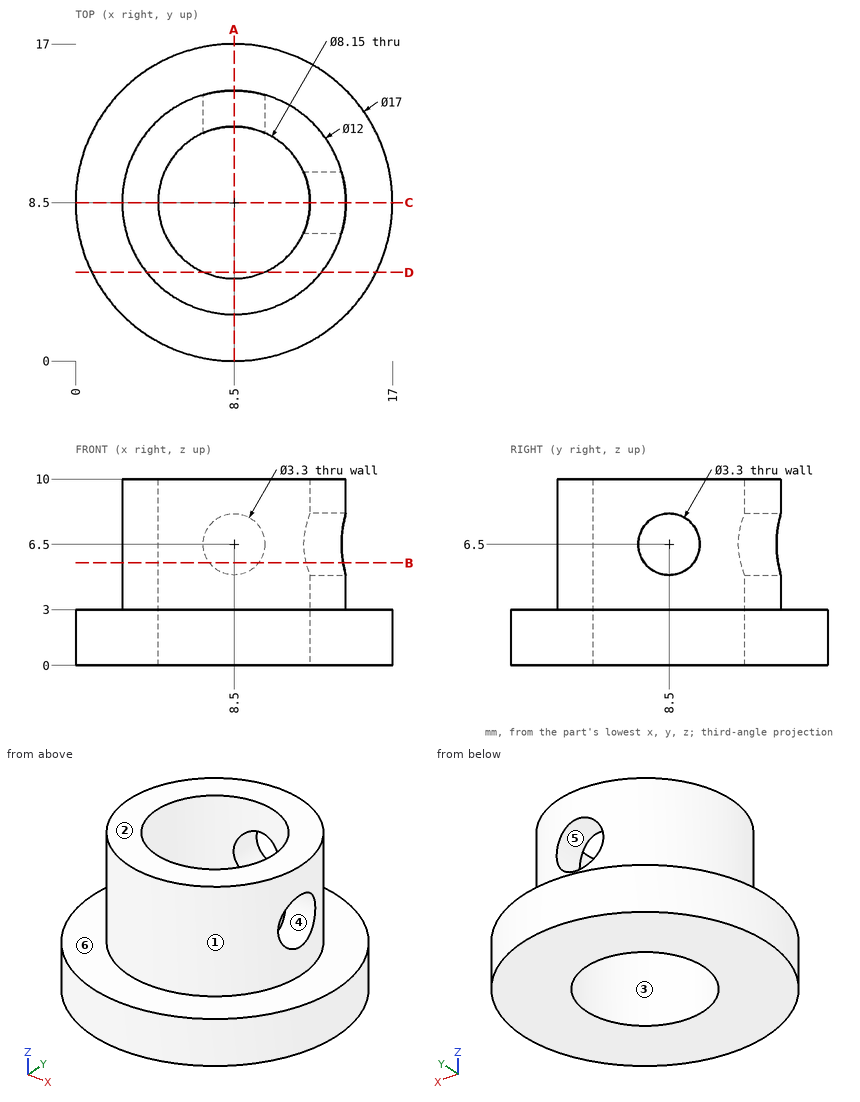
Answer from the drawing. Dimensions are ordinates in mm from the lowest x, y and z of the part. A direction names the side the tool comes from. Round coordinates to 2 decimals unless told otherwise and drop trailing zeros. Order: outer loops, then holes, each group sorted by start corner. A loop starts at its lowest first (then second) coordinate and runs counter-clockwise, first axis right, second up.
1) For the marked faces 4, 5 and 6, determine the directions among +Z, -Z, +X, -X, +Y, -Y from which every point of the face is accessible in a straight line to the end or side of a thin tool.
2) Flat-ended cylindrical pins translate along their axes: pin 1 (3 mm diameter, centred on x = 9.5, z = 8.5, fed in from +Y); pin 2 (1.5 mm diameter, centred on y = 6.5, z = 1.5, fed in from -X); pin 3 (4.5 mm diameter, centred on y = 8.5, z = 6.5, fed in from -X). Find the tip coordinate at first contact, or state that the pin passes through.
3) The part is cut by section D-D on y = 4.75. Write down the section's boundary in (x, z), plus the area to 3 significant figures.
4) The mould has two halves that part along Y. Classify the marked faces 1, 2 and 3: released by +Y, released by -Y, zero draft, split by the parting line, or undercut.
5) Straight lines are drawn through the part: L1, parallel to Z at x = 13.05, y = 8.5; L2, parallel to Y at x = 8.5, z = 8.25 (3 decimals); L3, parallel to Z at x = 9.5, y = 14.5. For each, find the intervals that lie inside material, in ascending order.
6) The part is cut by section B-B on z = 5.5. Write down the section's boundary in (x, y) (3 decimals), plus the area to 3 significant figures.
7) The part is cut by section A-A on x = 8.5. Write down the section's boundary in (y, z) (3 decimals).
Resolved:
1. face 4: +X
1. face 5: +Y
1. face 6: +Z
2. pin 1: stops at y = 14.5
2. pin 2: stops at x = 0.09
2. pin 3: stops at x = 2.5
3. outline: (0.87, 0) - (6.91, 0) - (6.91, 10) - (3.82, 10) - (3.82, 3) - (0.87, 3) - close; (10.09, 0) - (16.13, 0) - (16.13, 3) - (13.18, 3) - (13.18, 10) - (10.09, 10) - close
3. area: 79.4 mm2
4. face 1: split by the parting line
4. face 2: zero draft
4. face 3: undercut
5. L1: z = 0 to 4.85, 8.15 to 10
5. L2: y = 2.5 to 4.425, 12.575 to 14.5
5. L3: z = 0 to 3
6. outline: (7.188, 12.358) - (7.188, 14.355) arc R6 ccw (long way) to (14.355, 7.188) - (12.358, 7.188) arc R4.075 cw (long way) to start; (9.812, 12.358) arc R4.075 cw to (12.358, 9.812) - (14.355, 9.812) arc R6 ccw to (9.812, 14.355) - close
6. area: 50.7 mm2
7. outline: (0, 0) - (4.425, 0) - (4.425, 10) - (2.5, 10) - (2.5, 3) - (0, 3) - close; (12.575, 0) - (17, 0) - (17, 3) - (14.5, 3) - (14.5, 4.85) - (12.575, 4.85) - close; (12.575, 8.15) - (14.5, 8.15) - (14.5, 10) - (12.575, 10) - close
